Here's the drawing with two shaded views (mm, measured from the low corner). I have some questions. A direction names the side the tool comes from. Coordinates: 2 decimals unless noted, no trailing zeros. Write each loop counter-clockwise with the first axis right and the second up, starting at its lowest first coordinate (ties: lowest second). Pieces come first, ordered by that corner, then holes. Notation, with made-up numbers: (6.25, 80.25) -> (50.25, 80.25) arc R33 ccw to (50.25, 112.25) -> close; hole circle Ø7 at (58, 77.5). An arc over 180 degrees is marked (long way). Use one line per item in the form item = value.
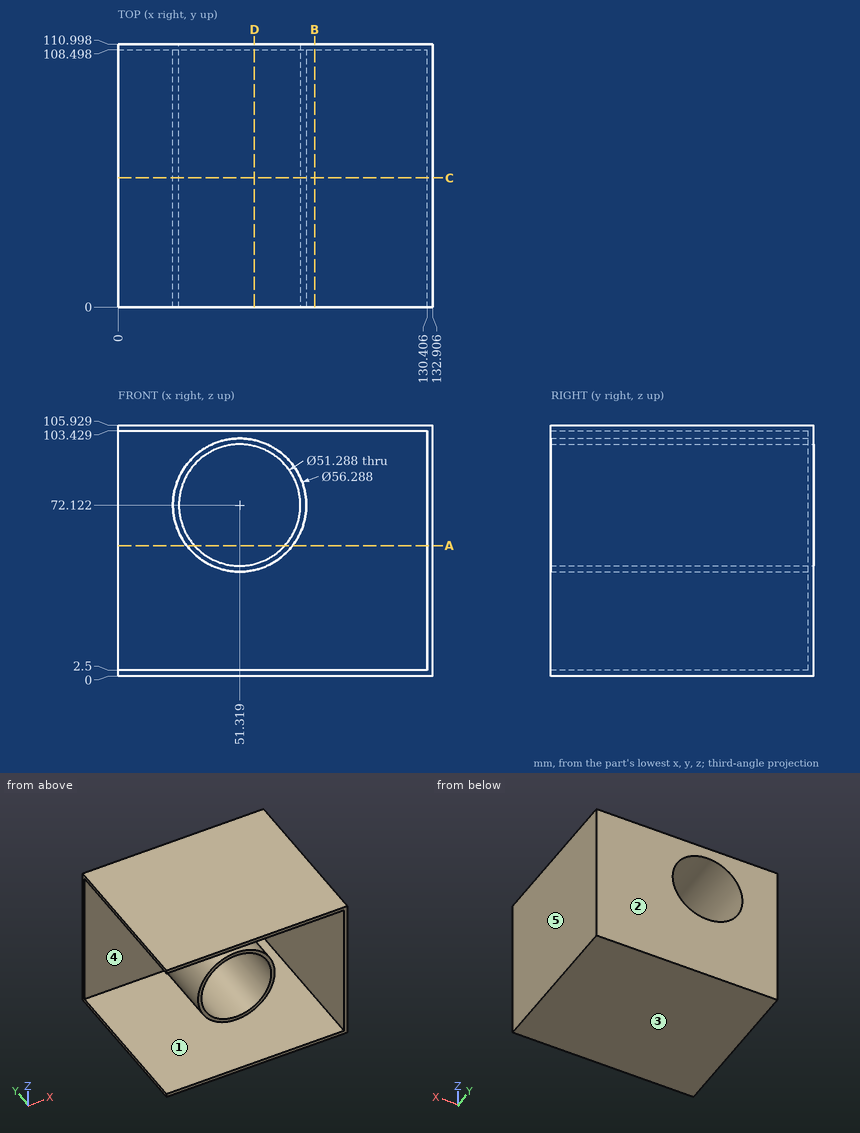
Q1. Thinking about a two-plate mould opening in Z: for the marked faces 1, 2 and 3, which applies, released by +Z, released by -Z, zero draft, split by the parting line, or undercut?
Return value:
face_1 = undercut
face_2 = zero draft
face_3 = released by -Z
Q2. Suppose I cut it at C-C (y = 54.5). Write out the boundary of the cut face in (x, z), then the cut area to 3 significant figures.
Return value:
outline = (0, 0) -> (132.91, 0) -> (132.91, 105.93) -> (0, 105.93) -> (0, 103.43) -> (130.41, 103.43) -> (130.41, 2.5) -> (0, 2.5) -> close; circle Ø56.29 at (51.32, 72.12); hole circle Ø51.29 at (51.32, 72.12)
area = 1,340 mm2
Q3. Will these pins go through, and if not, where does the flat tip stop? pin 1 (6 mm diameter, centred on x = 109, z = 26.5, fed in from -Y); pin 2 (3 mm diameter, centred on x = 112.5, y = 73.5, fed in from -Z); pin 3 (5 mm diameter, centred on y = 31, z = 56.5, fed in from -X).
Return value:
pin_1 = 108.5
pin_2 = 0
pin_3 = 26.42
Q4. Suppose I cut it at B-B (x = 83). Write out the boundary of the cut face in (y, z).
Return value:
outline = (0, 0) -> (111, 0) -> (111, 105.93) -> (0, 105.93) -> (0, 103.43) -> (108.5, 103.43) -> (108.5, 2.5) -> (0, 2.5) -> close
Q5. Suppose I cut it at A-A (z = 55). Write out the boundary of the cut face in (x, y) (1 decimal), then the cut area to 3 significant figures.
Return value:
outline = (0, 108.5) -> (29, 108.5) -> (29, 0) -> (32.2, 0) -> (32.2, 111) -> (0, 111) -> close; (70.4, 0) -> (73.7, 0) -> (73.7, 108.5) -> (130.4, 108.5) -> (130.4, 0) -> (132.9, 0) -> (132.9, 111) -> (70.4, 111) -> close
area = 1,210 mm2
Q6. Suppose I cut it at D-D (x = 57.5). Write out the boundary of the cut face in (y, z) (1 decimal), then the cut area to 3 significant figures.
Return value:
outline = (0, 0) -> (111, 0) -> (111, 47.2) -> (0, 47.2) -> (0, 44.7) -> (108.5, 44.7) -> (108.5, 2.5) -> (0, 2.5) -> close; (0, 97) -> (111, 97) -> (111, 105.9) -> (0, 105.9) -> (0, 103.4) -> (108.5, 103.4) -> (108.5, 99.6) -> (0, 99.6) -> close
area = 1,240 mm2
Q7. For the marked faces 4 and 5, which set-ups out of +Z, -Z, +X, -X, +Y, -Y let a thin tool reach every point of the face, with its end or its side?
Return value:
face_4 = -Y
face_5 = +Z, -Z, +X, +Y, -Y
Q8. If I drill on line 1 (Z direction, x = 50.5, y = 67); line 2 (Z direction, x = 52, y = 62); line 3 (Z direction, x = 123, y = 52), over which ranges is the centre line in solid material (lowest first)? Write a range as from..to.
Return value:
line_1 = 0..2.5, 43.99..46.49, 97.75..100.25, 103.43..105.93
line_2 = 0..2.5, 43.99..46.49, 97.76..100.26, 103.43..105.93
line_3 = 0..2.5, 103.43..105.93
